Can you work these out from the model? Positions are in its coordinate system, mm. Face numbers are marked on the shaded views. Give positions to 0.01 mm unless a question says otherwise; leave off trailing zeros. Write each loop counter-clockwise with the first axis right and the second up, starting at its lowest first coordinate (ties: lowest second). Pieces come first, ordered by that corner, then holes. Notation, with made-up numbers: M 86,-9 L 97,-9 A18 ccw 97,16 Z; hole C 54.5,77 d5. An arc over 180 degrees is marked long. Write each question's results on one line, items separated by ' | '.
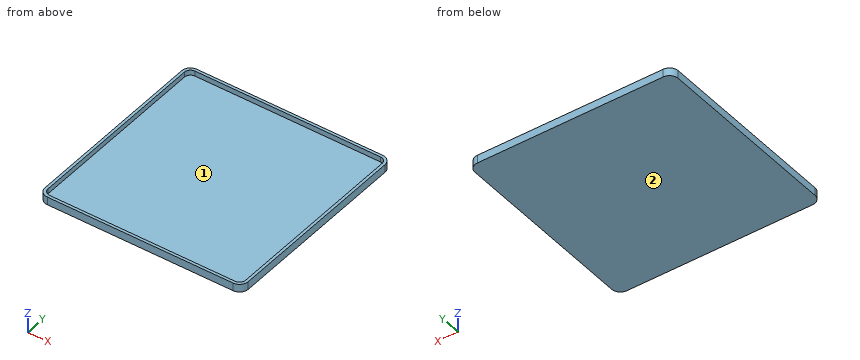
from build123d import *

# Parameters (mm, degrees)
SURFACE_EXTRUDE1_1_DEPTH = 3
THICKEN1_T1              = 1.6
THICKEN2_START           = -58.6
THICKEN2_OUTLINE_W       = 117.2
THICKEN2_OUTLINE_H       = 1.6
THICKEN2_DEPTH           = 117.2
FILLET2_R                = 5
FILLET3_R                = 3.5


# Read off the part's stored shape, not the designer's step: Thicken2
with BuildPart() as body_1:
    # Surface-Extrude1: a surface, the sketch's curves swept straight by 3 mm
    with BuildLine(Plane.XY, mode=Mode.PRIVATE) as surface_extrude1_1_path:
        Line((-57, 57), (57, 57))
        Line((57, 57), (57, -57))
        Line((57, -57), (-57, -57))
        Line((-57, -57), (-57, 57))
    surface_extrude1_1 = Shell.extrude(surface_extrude1_1_path.wire(), (0 * SURFACE_EXTRUDE1_1_DEPTH, 0 * SURFACE_EXTRUDE1_1_DEPTH, 1 * SURFACE_EXTRUDE1_1_DEPTH))
    add(Solid.thicken(surface_extrude1_1, THICKEN1_T1))

    # Thicken2 outline → Thicken2 (add)
    with BuildSketch(Plane.YZ.offset(THICKEN2_START)):
        with Locations((0, -0.8)):
            Rectangle(THICKEN2_OUTLINE_W, THICKEN2_OUTLINE_H)
    extrude(amount=THICKEN2_DEPTH)

    # Fillet2
    fillet2_edges = [body_1.edges().sort_by_distance(p)[0] for p in [
        (58.6, 58.6, 0.7),
        (-58.6, 58.6, 0.7),
        (58.6, -58.6, 0.7),
        (-58.6, -58.6, 0.7),
    ]]
    fillet(fillet2_edges, radius=FILLET2_R)

    # Fillet3
    fillet3_edges = [body_1.edges().sort_by_distance(p)[0] for p in [
        (57, 57, 1.5),
        (-57, 57, 1.5),
        (57, -57, 1.5),
        (-57, -57, 1.5),
    ]]
    fillet(fillet3_edges, radius=FILLET3_R)


solid = body_1.part
Item 1: I want a section at A-A, the plane z = 1.35. Please give me the cut outline in (x, y).
Geometry says:
outline: M -58.6,-53.6 A5 ccw -53.6,-58.6 L 53.6,-58.6 A5 ccw 58.6,-53.6 L 58.6,53.6 A5 ccw 53.6,58.6 L -53.6,58.6 A5 ccw -58.6,53.6 Z; hole M -57,-53.5 A3.5 ccw -53.5,-57 L 53.5,-57 A3.5 ccw 57,-53.5 L 57,53.5 A3.5 ccw 53.5,57 L -53.5,57 A3.5 ccw -57,53.5 Z
Item 2: I'm going to push a flat-ended pin straight in: pin 1 (8 mm diameter, centred on x = -20, y = -26, fed in from +Z). Where does the tip first touch, or does it pass through?
Geometry says:
pin 1: stops at z = 0
Item 3: I want a section at B-B, the plane y = 16.5. Please give me the cut outline in (x, z), and give its area (3 significant figures).
Geometry says:
outline: M -58.6,-1.6 L 58.6,-1.6 L 58.6,3 L 57,3 L 57,0 L -57,0 L -57,3 L -58.6,3 Z | area: 197 mm2
Item 4: Thinking about a two-plate mould opening in Y: for the marked faces 1 and 2, which applies, +Y half, -Y half, draft (parallel to the pull), parting line (faces both ways), or undercut?
Geometry says:
face 1: undercut | face 2: draft
Item 5: If I drill on line 1 (Y direction, x = -19.5, z = 1.8); line 2 (Z direction, x = 14, y = -38), over which ranges is the centre line in solid material (lowest first)? Write a range as from..to.
Geometry says:
line 1: y = -58.6..-57, 57..58.6 | line 2: z = -1.6..0
